Answer from the drawing. Dimensions are ordinates in mm from the lowest x, y and z of the part. Round coordinates to 2 decimals unless told otherwise and drop trailing zeros. Write each loop counter-clockwise with the first axis right and the second up, starting at its lowest first coordinate (ties: lowest second). Pieces come first, ordered by that corner, then holes. Notation, with made-up numbers: (67.5, -23) -> (90.5, -23) arc R23 ccw to (90.5, -9) -> close; hole circle Ø3 at (54.25, 76). An arc over 180 degrees is marked (long way). Return JSON: item names as keys, results as strings. Group by question number.
(1) A cutting plane is placed at B-B on z = 2.1. Give the vertices of the cut face in (x, y).
(2) A cutting plane is placed at C-C on x = 22.75. Give the vertices of the cut face in (y, z).
(3) A cutting plane is placed at A-A on x = 5.05. Give the vertices of the cut face in (y, z).
(4) Straight lines are drawn through the part: line 1 (Y direction, x = 22.75, z = 1.9); line 2 (Y direction, x = 14.65, z = 2.45); line 3 (X direction, y = 10.5, z = 2.75). For each, find the intervals that lie inside material, in ascending order.
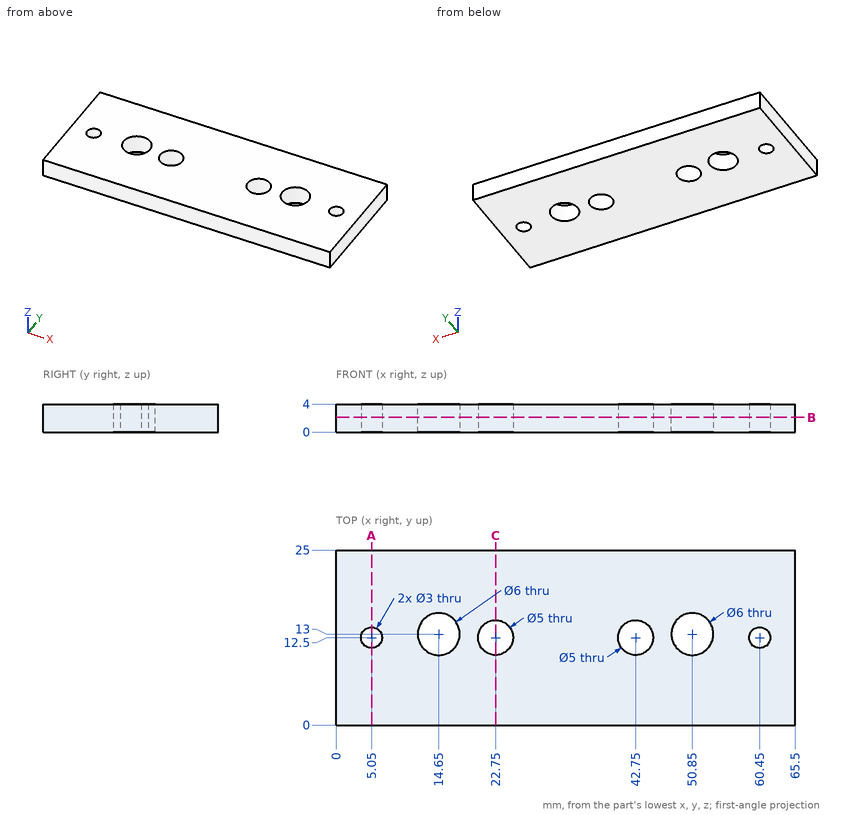
Checks:
{
 "1": {"outline": "(0, 0) -> (65.5, 0) -> (65.5, 25) -> (0, 25) -> close; hole circle Ø3 at (5.05, 12.5); hole circle Ø6 at (14.65, 13); hole circle Ø5 at (22.75, 12.5); hole circle Ø5 at (42.75, 12.5); hole circle Ø6 at (50.85, 13); hole circle Ø3 at (60.45, 12.5)"},
 "2": {"outline": "(0, 0) -> (10, 0) -> (10, 4) -> (0, 4) -> close; (15, 0) -> (25, 0) -> (25, 4) -> (15, 4) -> close"},
 "3": {"outline": "(0, 0) -> (11, 0) -> (11, 4) -> (0, 4) -> close; (14, 0) -> (25, 0) -> (25, 4) -> (14, 4) -> close"},
 "4": {"line 1": "y = 0 to 10, 15 to 25", "line 2": "y = 0 to 10, 16 to 25", "line 3": "x = 0 to 12.99, 16.31 to 21.25, 24.25 to 41.25, 44.25 to 49.19, 52.51 to 65.5"}
}
